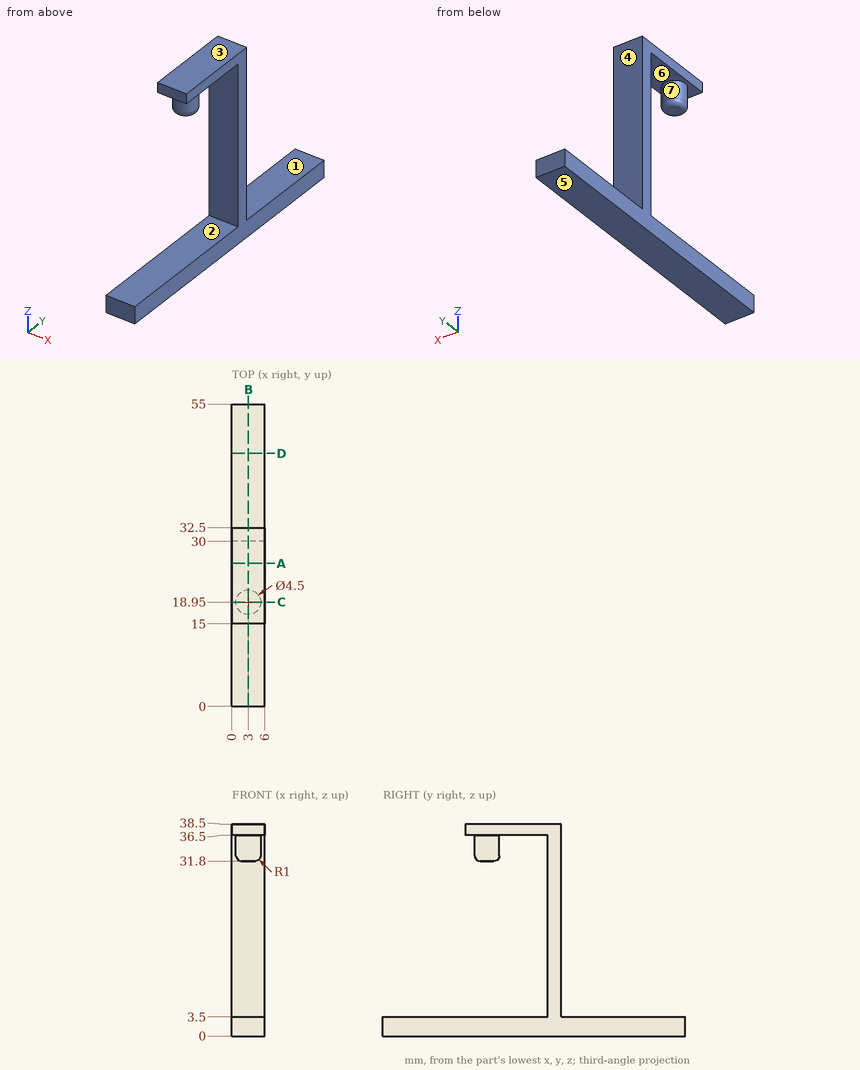
Verification items for this drawing (mm, ordinates from the low corner). A direction names the side the tool comes from. Give positions to 0.01 mm unless a question says otherwise; leave off trailing zeros. Loops run counter-clockwise (first coordinate to the right, second up) from the corner with the lowest first, then second, coordinate; pieces in that order, holes last.
1. Material ranges on probe 1 along Z at (x, y) = (5.1, 27.5); probe 2 along Z at (x, y) = (3.7, 37); probe 3 along Y at (x, z) = (3, 14), recorded low to high.
Derived:
probe 1: z = 0 to 3.5, 36.5 to 38.5
probe 2: z = 0 to 3.5
probe 3: y = 30 to 32.5
2. Go/stop test with flat-tipped pins: P1, Ø1.6, axis at x = 3.5, z = 37.5, coming from the -Y side; P2, Ø3, axis at x = 3.5, y = 8.5, coming from the +Z side. Record where each tip stops, or that it passes through.
Derived:
P1: stops at y = 15
P2: stops at z = 3.5
3. Cross-section at D-D on y = 46. Record the cut outline in (x, z), and give its area (3 significant figures).
Derived:
outline: (0, 0) - (6, 0) - (6, 3.5) - (0, 3.5) - close
area: 21.0 mm2
4. Tool access check on the marked faces 1, 2 and 3. Record the directions out of +Z, -Z, +X, -X, +Y, -Y that give a thin tool (end or side, any length) a straight path to the whole face; none if there is none.
Derived:
face 1: +Z, +X, -X, +Y
face 2: +X, -X, -Y
face 3: +Z, +X, -X, +Y, -Y
5. Cross-section at B-B on x = 3. Record the cut outline in (y, z), and give its area (3 significant figures).
Derived:
outline: (0, 0) - (55, 0) - (55, 3.5) - (32.5, 3.5) - (32.5, 38.5) - (15, 38.5) - (15, 36.5) - (16.7, 36.5) - (16.7, 32.8) arc R1 ccw to (17.7, 31.8) - (20.2, 31.8) arc R1 ccw to (21.2, 32.8) - (21.2, 36.5) - (30, 36.5) - (30, 3.5) - (0, 3.5) - close
area: 331 mm2
6. Cross-section at C-C on y = 18.95. Record the cut outline in (x, z), and give its area (3 significant figures).
Derived:
outline: (0, 0) - (6, 0) - (6, 3.5) - (0, 3.5) - close; (0, 36.5) - (0.75, 36.5) - (0.75, 32.8) arc R1 ccw to (1.75, 31.8) - (4.25, 31.8) arc R1 ccw to (5.25, 32.8) - (5.25, 36.5) - (6, 36.5) - (6, 38.5) - (0, 38.5) - close
area: 53.7 mm2
7. Cross-section at A-A on y = 26. Record the cut outline in (x, z).
Derived:
outline: (0, 0) - (6, 0) - (6, 3.5) - (0, 3.5) - close; (0, 36.5) - (6, 36.5) - (6, 38.5) - (0, 38.5) - close
8. Release check for a two-part mould opening along Z. For the marked faces 4, 5, 6 and 7 record: +Z half, -Z half, draft (parallel to the pull), parting line (faces both ways), or undercut.
Derived:
face 4: draft
face 5: -Z half
face 6: undercut
face 7: undercut
